```python
from build123d import *

# Parameters (mm, degrees)
SKETCH1_R           = 0.5
BOSS_EXTRUDE1_DEPTH = 15.5
SKETCH1_3_R         = 1.2
SKETCH1_3_R_2       = 0.5
BOSS_EXTRUDE2_DEPTH = 4.75
FILLET1_R           = 0.2
SKETCH2_R           = 0.85
BOSS_EXTRUDE3_DEPTH = 0.3
SKETCH4_W           = 0.471869861
SKETCH4_H           = 0.036263573
SKETCH5_W           = 0.976937104
SKETCH5_H           = 2.46
SKETCH6_R           = 0.5
BOSS_EXTRUDE5_DEPTH = 0.3


with BuildPart() as part:
    # Sketch1 → Boss-Extrude1 (new body)
    with BuildSketch(Plane.XY):
        Circle(SKETCH1_R)
    extrude(amount=BOSS_EXTRUDE1_DEPTH)



with BuildPart() as body_2:
    # Sketch1_3 → Boss-Extrude2 (new body)
    with BuildSketch(Plane.XY):
        Circle(SKETCH1_3_R)
        Circle(SKETCH1_3_R_2, mode=Mode.SUBTRACT)
    extrude(amount=-BOSS_EXTRUDE2_DEPTH)

    # Fillet1
    fillet1_edges = [body_2.edges().sort_by_distance(p)[0] for p in [
        (-1.2, 0, 0),
    ]]
    fillet(fillet1_edges, radius=FILLET1_R)


with BuildPart() as part_1:
    add(part.part)

    add(body_2.part)  # Boss-Extrude3 merges body 2
    # Sketch2 → Boss-Extrude3 (add)
    with BuildSketch(Plane.XY):
        Circle(SKETCH2_R)
    extrude(amount=BOSS_EXTRUDE3_DEPTH)

    # Sketch3 → Revolve1 (revolve)
    with BuildSketch(Plane(origin=(0, 0, 0), x_dir=(1, 0, 0), z_dir=(0, 1, 0)), mode=Mode.PRIVATE) as revolve1_sk:
        with BuildLine():
            Line((0.5, -15.5), (0, -15.5))
            Line((0, -15.5), (0, -16.08))
            ThreePointArc((0, -16.08), (0.247487373, -16.182512627), (0.35, -16.43))
            Line((0.35, -16.43), (0.5, -16.43))
            ThreePointArc((0.5, -16.43), (0.470461057, -16.26068847), (0.385334423, -16.111382075))
            Line((0.385334423, -16.111382075), (0.385334423, -15.967978567))
            Line((0.385334423, -15.967978567), (0.5, -15.967978567))
            Line((0.5, -15.967978567), (0.5, -15.793310987))
            Line((0.5, -15.793310987), (0.416056351, -15.793310987))
            ThreePointArc((0.416056351, -15.793310987), (0.437455238, -15.640767656), (0.5, -15.5))
        make_face()
    revolve(revolve1_sk.sketch.rotate(Axis((0, 0, 15.5), (0, 0, 1)), 180), axis=Axis((0, 0, 15.5), (0, 0, 1)))

    # Sketch4 → Revolve2 (revolve)
    with BuildSketch(Plane(origin=(0, 0, 0), x_dir=(1, 0, 0), z_dir=(0, 1, 0)), mode=Mode.PRIVATE) as revolve2_sk:
        with Locations((-0.235934931, -16.321868214)):
            Rectangle(SKETCH4_W, SKETCH4_H)
    revolve(revolve2_sk.sketch.rotate(Axis((0, 0, 15.5), (0, 0, 1)), 180), axis=Axis((0, 0, 15.5), (0, 0, 1)))

    # Sketch5 → Cut-Revolve1 (revolve, cut)
    with BuildSketch(Plane(origin=(0, 0, 0), x_dir=(1, 0, 0), z_dir=(0, 1, 0))):
        with Locations((-0.755461177, -14.27)):
            Rectangle(SKETCH5_W, SKETCH5_H)
    revolve(axis=Axis((0, 0, 15.5), (0, 0, 1)), mode=Mode.SUBTRACT)

    # Sketch6 → Boss-Extrude5 (add)
    with BuildSketch(Plane(origin=(0, 0, -4.75), x_dir=(-1, 0, 0), z_dir=(0, 0, -1))):
        Circle(SKETCH6_R)
    extrude(amount=-BOSS_EXTRUDE5_DEPTH)


solid = part_1.part
```
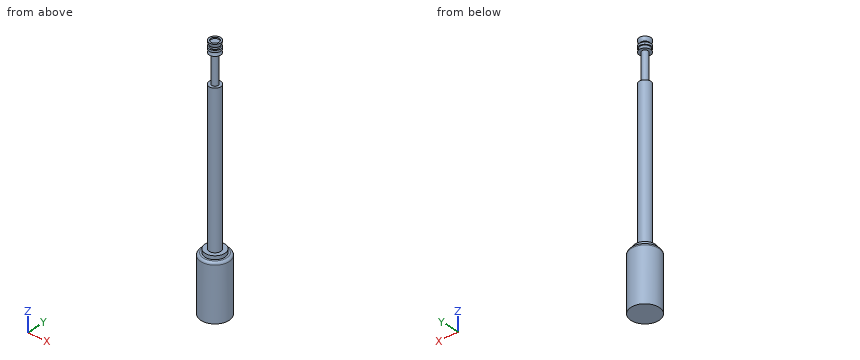
Can you work these out from the model? Positions are in its coordinate system, mm. Coordinates: 2 decimals unless noted, no trailing zeros. Loops run counter-clockwise (first coordinate to the right, second up) from the corner with the lowest first, then second, coordinate; pieces in that order, holes last.
1) Imagine slicing it at C-C on x = 0. State how many separate pieces and enclosed holes the cut face has, plus the area to 3 significant figures.
2) For pin 1 (1 mm diameter, centred on x = 0, y = 0, fed in from +Z); pin 2 (0.5 mm diameter, centred on x = 0, y = 0, fed in from +Z), each with a flat end and sliding along its axis, tell me the tip position at first contact or that it passes through.
3) I need wall thicknesses on probe 1 along Y at (x, z) = (0, -1.7); probe 2 along Z at (x, y) = (-0.9, -0.1); probe 3 along Z at (x, y) = (0, 0.7). Which ranges of each line are inside material? Lowest first, please.
4) Imagine slicing it at B-B on z = 14. List the corners of the cut face in (x, y) for me, plus the area to 3 significant figures.
5) Imagine slicing it at A-A on z = -3. List the corners of the cut face in (x, y) for me, plus the area to 3 significant figures.
Completed:
1. separate pieces: 1
1. enclosed holes: 2
1. area: 22.2 mm2
2. pin 1: stops at z = 16.43
2. pin 2: stops at z = 16.34
3. probe 1: y = -1.2 to -0.5, 0.5 to 1.2
3. probe 2: z = -4.75 to 0
3. probe 3: z = -4.75 to 0.3
4. outline: circle Ø0.53 at (0, 0)
4. area: 0.224 mm2
5. outline: circle Ø2.4 at (0, 0); hole circle Ø1 at (0, 0)
5. area: 3.74 mm2
